```python
from build123d import *

# Parameters (mm, degrees)
SKETCH1_W                 = 110
SKETCH1_H                 = 85
BASE_DEPTH                = 25
FILLET1_R                 = 5
SKETCH2_W                 = 96.5
SKETCH2_H                 = 73
BASKET_DEPTH              = 19
SKETCH3_W                 = 4
SKETCH3_H                 = 6
WIRE_CHANNEL_DEPTH        = 19
WIRE_CHANNEL_ROUNDING_R   = 1
SWITCH_CUT_OUT_REACH      = 106.283
SKETCH5_W                 = 17
SKETCH5_H                 = 15
SWITCH_CUT_OUT_ROUNDING_R = 3
SKETCH14_R                = 1.75
CORNER_HOLES_DEPTH        = 74.866433513
BOTTOM_NUT_CUT_OUT_DEPTH  = 3


with BuildPart() as part:
    # Sketch1 → Base (new body)
    with BuildSketch(Plane(origin=(0, 0, 0), x_dir=(1, 0, 0), z_dir=(0, 1, 0))):
        Rectangle(SKETCH1_W, SKETCH1_H)
    extrude(amount=BASE_DEPTH)

    # Fillet1
    fillet1_edges = [part.edges().sort_by_distance(p)[0] for p in [
        (55, 12.5, 42.5),
        (-55, 12.5, 42.5),
        (-55, 12.5, -42.5),
        (55, 12.5, -42.5),
    ]]
    fillet(fillet1_edges, radius=FILLET1_R)

    # Sketch2 → Basket (cut)
    with BuildSketch(Plane(origin=(0, 25, 0), x_dir=(1, 0, 0), z_dir=(0, 1, 0))):
        Rectangle(SKETCH2_W, SKETCH2_H)
    extrude(amount=-BASKET_DEPTH, mode=Mode.SUBTRACT)

    # Sketch3 → Wire Channel (cut)
    with BuildSketch(Plane(origin=(0, 25, 0), x_dir=(1, 0, 0), z_dir=(0, 1, 0))):
        with Locations((-15, -36.5)):
            Rectangle(SKETCH3_W, SKETCH3_H)
    extrude(amount=-WIRE_CHANNEL_DEPTH, mode=Mode.SUBTRACT)

    # Wire Channel Rounding
    wire_channel_rounding_edges = [part.edges().sort_by_distance(p)[0] for p in [
        (-17, 15.5, 39.5),
        (-13, 15.5, 39.5),
    ]]
    fillet(wire_channel_rounding_edges, radius=WIRE_CHANNEL_ROUNDING_R)

    # Sketch5 → Switch Cut-out (cut, up to next)
    with BuildSketch(Plane.XY.offset(42.5), mode=Mode.PRIVATE) as switch_cut_out_sk1:
        with Locations((-34.75, 17.5)):
            Rectangle(SKETCH5_W, SKETCH5_H)
    switch_cut_out_tool1 = extrude(switch_cut_out_sk1.sketch, amount=-SWITCH_CUT_OUT_REACH, mode=Mode.PRIVATE) & part.part
    add(switch_cut_out_tool1.solids().sort_by_distance((-34.75, 17.5, 42.5))[0], mode=Mode.SUBTRACT)

    # Switch Cut-out Rounding
    switch_cut_out_rounding_edges = [part.edges().sort_by_distance(p)[0] for p in [
        (-43.25, 17.5, 42.5),
        (-34.75, 10, 42.5),
        (-26.25, 17.5, 42.5),
    ]]
    fillet(switch_cut_out_rounding_edges, radius=SWITCH_CUT_OUT_ROUNDING_R)

    # Sketch14 → Corner Holes (cut, through all)
    with BuildSketch(Plane(origin=(0, 25, 0), x_dir=(1, 0, 0), z_dir=(0, 1, 0))):
        with Locations(Location((-50.892766953, 38.767766953, 0), (0, 0, 270))):
            Circle(SKETCH14_R)
        with Locations(Location((50.892766953, 38.767766953, 0), (0, 0, 270))):
            Circle(SKETCH14_R)
        with Locations(Location((50.892766953, -38.767766953, 0), (0, 0, 270))):
            Circle(SKETCH14_R)
        with Locations(Location((-50.892766953, -38.767766953, 0), (0, 0, 270))):
            Circle(SKETCH14_R)
    extrude(amount=-CORNER_HOLES_DEPTH, mode=Mode.SUBTRACT)

    # Sketch15 → Bottom Nut Cut-out (cut)
    with BuildSketch(Plane.XZ):
        Polygon((-50.64101323, 42.388469214), (-52.178282629, 43.416097239), (-55.727023172, 38.10739593), (-54.143831126, 37.15203238), (-51.13140477, 35.13829702), (-47.868872697, 36.746365575), (-47.630234881, 40.375835508), align=None)
        Polygon((50.595962101, 42.39294376), (52.091508492, 43.427758232), (55.676210978, 38.247033564), (54.180664587, 37.212219092), (51.189571805, 35.142590146), (47.901674171, 36.698138008), (47.604869319, 40.323314814), align=None)
        Polygon((54.167766953, -36.699113605), (55.742766953, -37.608440279), (52.313760602, -43.547653498), (50.738760602, -42.638326824), (47.463760602, -40.747504693), (47.463760602, -36.788029213), (50.892766953, -34.808291473), align=None)
        Polygon((-53.9527362, -36.801402743), (-55.569189191, -37.634817242), (-52.682156679, -43.23437466), (-51.065703688, -42.400960161), (-47.832797706, -40.734131163), (-47.65986097, -37.100937955), (-50.719830218, -35.134573745), align=None)
    extrude(amount=-BOTTOM_NUT_CUT_OUT_DEPTH, mode=Mode.SUBTRACT)


solid = part.part
```
For this review, take the finished solid that the model builds, in its own axes (mm). A direction names the side the tool comes from. Round coordinates to 2 decimals unless told otherwise and drop trailing zeros. Write each loop counter-clockwise with the first axis right and the second up, starting at its lowest first coordinate (ties: lowest second). Pieces come first, ordered by that corner, then holes. Notation, with made-up numbers: (54, 76) - (68, 76) arc R36 ccw to (68, 110) - close; hole circle Ø7 at (-4.75, 65). An arc over 180 degrees is marked (long way). Answer as a JSON object with one key per item and string values.
1. For pin 1 Ø2 at (x, z) = (-53, 39) entering from -Y; pin 2 Ø3.5 at (x, z) = (-31, 38.5) entering from +Y; pin 3 Ø1.5 at (y, z) = (1, -39) entering from +X; pin 4 Ø3 at (x, z) = (-50.89, 38.77) entering from +Y, all flat-tipped, find the tip position at first contact; note any pin that passes through.
Response values:
{"pin 1": "stops at y = 3", "pin 2": "stops at y = 10", "pin 3": "stops at x = 47.46", "pin 4": "passes through"}
2. Tool access review of faces 1 (the face through (-26.25, 17, 38)), 2 (the face through (-47.75, 1.48, 38.54)), 3 (the face through (-52.66, 1.48, 36.16)): name each direction out of +Z, -Z, +X, -X, +Y, -Y from which nothing blocks a thin tool from reaching the whole face with its end or side.
Response values:
{"face 1": "+Z, +Y", "face 2": "-Y", "face 3": "+Z, -Y"}
3. We need section B-B on x = -41.5. Give the boundary of the cut face in (y, z), then the cut area to 3 significant figures.
Response values:
{"outline": "(0, -42.5) - (25, -42.5) - (25, -36.5) - (6, -36.5) - (6, 36.5) - (10, 36.5) - (10, 39.5) arc R3 ccw to (7, 42.5) - (0, 42.5) - close", "area": "646 mm2"}
4. We need section A-A on z = -12.5. Give the boundary of the cut face in (x, y).
Response values:
{"outline": "(-55, 0) - (55, 0) - (55, 25) - (48.25, 25) - (48.25, 6) - (-48.25, 6) - (-48.25, 25) - (-55, 25) - close"}
5. Draft analysis for pull direction X (two halves, no side actions). For faces 4 (the face through (-1, 0, -1)), 5 (the face through (49.57, 1.48, 35.91)), 6 (the face through (-53.57, 12.68, -41)), state which applies: +X half, -X half, draft (parallel to the pull), parting line (faces both ways), or undercut.
Response values:
{"face 4": "draft", "face 5": "undercut", "face 6": "-X half"}
6. We need section D-D on y = 8.5. Give the boundary of the cut face in (x, z).
Response values:
{"outline": "(-55, -37.5) arc R5 ccw to (-50, -42.5) - (50, -42.5) arc R5 ccw to (55, -37.5) - (55, 37.5) arc R5 ccw to (50, 42.5) - (-23.25, 42.5) arc R3 ccw to (-24.75, 42.1) - (-44.75, 42.1) arc R3 ccw to (-46.25, 42.5) - (-50, 42.5) arc R5 ccw to (-55, 37.5) - close; hole circle Ø3.5 at (-50.89, -38.77); hole circle Ø3.5 at (-50.89, 38.77); hole (-48.25, -36.5) - (48.25, -36.5) - (48.25, 36.5) - (-13, 36.5) - (-13, 38.5) arc R1 ccw to (-14, 39.5) - (-16, 39.5) arc R1 ccw to (-17, 38.5) - (-17, 36.5) - (-48.25, 36.5) - close; hole circle Ø3.5 at (50.89, -38.77); hole circle Ø3.5 at (50.89, 38.77)"}
7. To check wall thickness, follow line 1 along X through (y, z) = (17.5, -19); line 2 along Z through (x, y) = (8, 16); line 3 along Y through (x, z) = (-16.5, -10.5). State the ranges of each line that lie inside material, in increasing order.
Response values:
{"line 1": "x = -55 to -48.25, 48.25 to 55", "line 2": "z = -42.5 to -36.5, 36.5 to 42.5", "line 3": "y = 0 to 6"}
8. We need section C-C on y = 14.75. Give the boundary of the cut face in (x, z), then the cut area to 3 significant figures.
Response values:
{"outline": "(-55, -37.5) arc R5 ccw to (-50, -42.5) - (50, -42.5) arc R5 ccw to (55, -37.5) - (55, 37.5) arc R5 ccw to (50, 42.5) - (-23.25, 42.5) arc R3 ccw to (-26.25, 39.5) - (-26.25, 36.5) - (-17, 36.5) - (-17, 38.5) arc R1 cw to (-16, 39.5) - (-14, 39.5) arc R1 cw to (-13, 38.5) - (-13, 36.5) - (48.25, 36.5) - (48.25, -36.5) - (-48.25, -36.5) - (-48.25, 36.5) - (-43.25, 36.5) - (-43.25, 39.5) arc R3 ccw to (-46.25, 42.5) - (-50, 42.5) arc R5 ccw to (-55, 37.5) - close; hole circle Ø3.5 at (-50.89, -38.77); hole circle Ø3.5 at (-50.89, 38.77); hole circle Ø3.5 at (50.89, -38.77); hole circle Ø3.5 at (50.89, 38.77)", "area": "2,130 mm2"}
